from build123d import *

# Parameters (mm, degrees)
F1_DEPTH = 200
F2_W     = 10.593976
F2_H     = 10
F3_DEPTH = 467


with BuildPart() as f1:
    # F0 (on Top) → F1 (new body)
    with BuildSketch(Plane.XY):
        Polygon((40, 297.683151), (274.538241, 0), (300, 0), (40, 330), align=None)
    extrude(amount=F1_DEPTH)

    # F2 (on Right) → F3 (cut)
    with BuildSketch(Plane.YZ):
        with BuildLine():
            ThreePointArc((0, 170), (2.928932, 177.071068), (10, 180))
            Line((10, 180), (-16.794052, 180))
            Line((-16.794052, 180), (-16.794052, 171.051905))
            Line((-16.794052, 171.051905), (0, 170))
        make_face()
        with Locations((-5.296988, 25)):
            Rectangle(F2_W, F2_H)
        with BuildLine():
            Line((80, 30), (80, 170))
            ThreePointArc((80, 170), (77.071068, 177.071068), (70, 180))
            Line((70, 180), (10, 180))
            ThreePointArc((10, 180), (2.928932, 177.071068), (0, 170))
            Line((0, 170), (0, 100))
            Line((0, 100), (0, 30))
            ThreePointArc((0, 30), (2.928932, 22.928932), (10, 20))
            Line((10, 20), (70, 20))
            ThreePointArc((70, 20), (77.071068, 22.928932), (80, 30))
        make_face()
        with BuildLine():
            Line((0, 20), (10, 20))
            ThreePointArc((10, 20), (2.928932, 22.928932), (0, 30))
            Line((0, 30), (0, 20))
        make_face()
    extrude(amount=F3_DEPTH, mode=Mode.SUBTRACT)


solid = f1.part
Read the model definition and answer for the solid it produces. Units are mm, in the model's axes. A direction names the side the tool comes from. Give positions to 0.01 mm unless a question says otherwise; leave off trailing zeros. Write each loop counter-clockwise with the first axis right and the second up, starting at its lowest first coordinate (ties: lowest second). Pieces come first, ordered by that corner, then holes. Notation, with made-up numbers: (69.25, 50) - (99.25, 50) arc R24 cw to (99.25, 77) - close; hole circle Ø5 at (88, 45). An arc over 180 degrees is marked (long way). Answer in a Markdown table with one row per item. Add a question column.
Item 1: Section A-A, the plane z = 163.5 is taken. Write down the section's boundary in (x, y), and give its area (3 significant figures).
Item 2: Find the intervals of material crossed by L1, parallel to Y at x = 234, z = 88.5; L2, parallel to Y at x = 59, z = 59; L3, parallel to X at y = 74.5, z = 188.5, in increasing order.
Item 3: Determine the mould class of faces 1 (the face through (160, 154, 200)), 2 (the face through (160, 154, 0)), 3 (the face through (224, 80, 99)), 4 (the face through (227.94, 77.15, 176.99)) for opening direction Z: pulls with the +Z half, pulls with the -Z half, needs draft (parallel to the pull), parting line crosses it, or undercut.
Item 4: Flat-ended cylindrical pins translate along their axes: P1, Ø6, axis at y = 269.5, z = 102, coming from the +X side; P2, Ø1, axis at y = 124.5, z = 82, coming from the +X side; P3, Ø5, axis at x = 119, z = 71, coming from the -Y side. Find the tip coordinate at first contact, or state that the pin passes through.
Item 5: A tool of negligible diameter and unlimited length cuts with its end or side. For faces 5 (the face through (227.94, 76.99, 22.85)), 6 (the face through (40, 314, 99)), from which of +Z, -Z, +X, -X, +Y, -Y can it reach the whole face along a straight path? Write none if from no direction.
Item 6: Section B-B, the plane x = 155 is taken. Write down the section's boundary in (y, z).
Recorded:
| question | item | result |
|---|---|---|
| 1 | outline | (40, 297.68) - (211.51, 80) - (236.97, 80) - (40, 330) - close |
| 1 | area | 5,950 mm2 |
| 2 | L1 | y = 80 to 83.77 |
| 2 | L2 | y = 273.57 to 305.88 |
| 2 | L3 | x = 215.84 to 241.3 |
| 3 | face 1 | pulls with the +Z half |
| 3 | face 2 | pulls with the -Z half |
| 3 | face 3 | undercut |
| 3 | face 4 | undercut |
| 4 | P1 | stops at x = 90.03 |
| 4 | P2 | stops at x = 202.3 |
| 4 | P3 | stops at y = 194.24 |
| 5 | face 5 | +X, -X, -Y |
| 5 | face 6 | +Z, -Z, -X, +Y, -Y |
| 6 | outline | (151.72, 0) - (184.04, 0) - (184.04, 200) - (151.72, 200) - close |
